Work out the finished part from the listing and answer in its coordinate system (mm). A direction names the side the tool comes from. Round coordinates to 2 decimals unless told otherwise and drop trailing zeros. Loops run counter-clockwise (first coordinate to the right, second up) from the corner with the lowest first, then second, coordinate; pieces in that order, holes last. Notation, with made-up numbers: (8.25, 74) -> (32.25, 74) arc R34 ccw to (32.25, 113) -> close; hole circle Ø10 at (56.25, 60). An arc over 180 degrees is marked (long way). Write item = value, one per line. Start each with the question number.
```python
from build123d import *

# Parameters (mm, degrees)
F0_W     = 104
F0_H     = 55
F1_DEPTH = 2
F2_DEPTH = 25
F3_SIZE  = 2


with BuildPart() as f1:
    # F0 (on Top) → F1 (new body)
    with BuildSketch(Plane.XY):
        Rectangle(F0_W, F0_H)
    extrude(amount=F1_DEPTH)

    # F0 (on Top) → F2 (join)
    with BuildSketch(Plane.XY):
        Polygon((52, 27.5), (52, -27.5), (54.2, -27.5), (54.2, 29.7), (-54.2, 29.7), (-54.2, -27.5), (-52, -27.5), (-52, 27.5), align=None)
    extrude(amount=F2_DEPTH)

    # F3
    f3_edges = [f1.edges().sort_by_distance(p)[0] for p in [
        (54.2, 29.7, 12.5),
        (-54.2, 29.7, 12.5),
        (-54.2, -27.5, 12.5),
        (54.2, -27.5, 12.5),
    ]]
    chamfer(f3_edges, length=F3_SIZE)


solid = f1.part
```
Item 1: The mould has two halves that part along X. Classify faces 1 (the flat face through (53.2, -26.5, 12.3)), 2 (the flat face through (-53.2, -26.5, 12.3)), 3 (the flat face through (0, -27.5, 1)), 4 (the flat face through (52, 0, 13)): pulls with the +X half, pulls with the -X half, needs draft (parallel to the pull), parting line crosses it, or undercut.
Item 2: Section C-C (x = -26) is taken. Determine the outline of the cut face in (y, z).
Item 3: Section B-B (y = -18.5) is taken. Determine the outline of the cut face in (x, z).
Item 4: Find the intervals of material crossed by line 1 along X through (y, z) = (15, 14.5); line 2 along Z through (x, y) = (-22.5, 19); line 3 along Y through (x, z) = (-1, 3.75), in increasing order. Write a range as [from, to].
Item 5: Flat-ended cylindrical pins translate along their axes: pin 1 (2 mm diameter, centred on x = 36.5, y = 1, fed in from +Z); pin 2 (2 mm diameter, centred on x = -40, z = 7, fed in from -Y); pin 3 (1.5 mm diameter, centred on x = 5.5, y = 0.5, fed in from -Z). Find the tip coordinate at first contact, or state that the pin passes through.
Item 6: Section A-A (z = 13) is taken. Determine the outline of the cut face in (x, y), then the cut area to 3 significant figures.
Item 7: A tool of negligible diameter and unlimited length cuts with its end or side. For faces 5 (the flat face through (-53.2, 28.7, 12.3)), 6 (the flat face through (-1, 0, 2)), from which of +Z, -Z, +X, -X, +Y, -Y can it reach the whole face along a straight path? Write none if from no direction.
Worked answers:
q1.face_1 = pulls with the +X half
q1.face_2 = pulls with the -X half
q1.face_3 = needs draft
q1.face_4 = undercut
q2.outline = (-27.5, 0) -> (29.7, 0) -> (29.7, 25) -> (27.5, 25) -> (27.5, 2) -> (-27.5, 2) -> close
q3.outline = (-54.2, 0) -> (54.2, 0) -> (54.2, 25) -> (52, 25) -> (52, 2) -> (-52, 2) -> (-52, 25) -> (-54.2, 25) -> close
q4.line_1 = [-54.2, -52], [52, 54.2]
q4.line_2 = [0, 2]
q4.line_3 = [27.5, 29.7]
q5.pin_1 = 2
q5.pin_2 = 27.5
q5.pin_3 = 0
q6.outline = (-54.2, -25.5) -> (-52.2, -27.5) -> (-52, -27.5) -> (-52, 27.5) -> (52, 27.5) -> (52, -27.5) -> (52.2, -27.5) -> (54.2, -25.5) -> (54.2, 27.7) -> (52.2, 29.7) -> (-52.2, 29.7) -> (-54.2, 27.7) -> close
q6.area = 472 mm2
q7.face_5 = +Z, -Z, -X, +Y
q7.face_6 = +Z, -Y
